```python
from build123d import *

# Parameters (mm, degrees)
EXTRUDE_1_DEPTH     = 5
CUT_EXTRUDE_1_DEPTH = 5
SKETCH_3_R          = 1.65
CUT_EXTRUDE_2_DEPTH = 10
SKETCH_4_R          = 11.2
SKETCH_4_R_2        = 11
SKETCH_4_R_3        = 1.65
SKETCH_4_R_4        = 1.6
CUT_EXTRUDE_3_DEPTH = 10
FILLET_1_R          = 15


with BuildPart() as part:
    # 草图1 → 凸台-拉伸1 (new body)
    with BuildSketch(Plane.XY):
        Polygon((65, 65), (65, 0), (195, 0), (195, 65), (260, 65), (260, 195), (195, 195), (195, 260), (65, 260), (65, 195), (0, 195), (0, 65), align=None)
    extrude(amount=EXTRUDE_1_DEPTH)

    # 草图2 → 切除-拉伸1 (cut)
    with BuildSketch(Plane(origin=(0, 0, 0), x_dir=(-1, 0, 0), z_dir=(0, 0, -1))):
        with BuildLine():
            Line((-106.8, 12.1), (-77, 12.1))
            ThreePointArc((-77, 12.1), (-74.9, 10), (-77, 7.9))
            Line((-77, 7.9), (-106.8, 7.9))
            ThreePointArc((-106.8, 7.9), (-108.9, 10), (-106.8, 12.1))
        make_face()
        with BuildLine():
            Line((-106.8, 42.1), (-77, 42.1))
            ThreePointArc((-77, 42.1), (-74.9, 40), (-77, 37.9))
            Line((-77, 37.9), (-106.8, 37.9))
            ThreePointArc((-106.8, 37.9), (-108.9, 40), (-106.8, 42.1))
        make_face()
        with BuildLine():
            Line((-153.2, 12.1), (-183, 12.1))
            ThreePointArc((-183, 12.1), (-185.1, 10), (-183, 7.9))
            Line((-183, 7.9), (-153.2, 7.9))
            ThreePointArc((-153.2, 7.9), (-151.1, 10), (-153.2, 12.1))
        make_face()
        with BuildLine():
            Line((-153.2, 42.1), (-183, 42.1))
            ThreePointArc((-183, 42.1), (-185.1, 40), (-183, 37.9))
            Line((-183, 37.9), (-153.2, 37.9))
            ThreePointArc((-153.2, 37.9), (-151.1, 40), (-153.2, 42.1))
        make_face()
        with BuildLine():
            Line((-106.8, 247.9), (-77, 247.9))
            ThreePointArc((-77, 247.9), (-74.9, 250), (-77, 252.1))
            Line((-77, 252.1), (-106.8, 252.1))
            ThreePointArc((-106.8, 252.1), (-108.9, 250), (-106.8, 247.9))
        make_face()
        with BuildLine():
            Line((-106.8, 217.9), (-77, 217.9))
            ThreePointArc((-77, 217.9), (-74.9, 220), (-77, 222.1))
            Line((-77, 222.1), (-106.8, 222.1))
            ThreePointArc((-106.8, 222.1), (-108.9, 220), (-106.8, 217.9))
        make_face()
        with BuildLine():
            Line((-153.2, 247.9), (-183, 247.9))
            ThreePointArc((-183, 247.9), (-185.1, 250), (-183, 252.1))
            Line((-183, 252.1), (-153.2, 252.1))
            ThreePointArc((-153.2, 252.1), (-151.1, 250), (-153.2, 247.9))
        make_face()
        with BuildLine():
            Line((-153.2, 217.9), (-183, 217.9))
            ThreePointArc((-183, 217.9), (-185.1, 220), (-183, 222.1))
            Line((-183, 222.1), (-153.2, 222.1))
            ThreePointArc((-153.2, 222.1), (-151.1, 220), (-153.2, 217.9))
        make_face()
    extrude(amount=-CUT_EXTRUDE_1_DEPTH, mode=Mode.SUBTRACT)

    # 草图3 → 切除-拉伸2 (cut)
    with BuildSketch(Plane.XY.offset(5)):
        with Locations((250, 185)):
            Circle(SKETCH_3_R)
        with Locations((250, 75)):
            Circle(SKETCH_3_R)
        with Locations((10, 75)):
            Circle(SKETCH_3_R)
        with Locations((10, 185)):
            Circle(SKETCH_3_R)
        with Locations((130, 75)):
            Circle(SKETCH_3_R)
        with Locations((130, 185)):
            Circle(SKETCH_3_R)
    extrude(amount=-CUT_EXTRUDE_2_DEPTH, mode=Mode.SUBTRACT)

    # 草图4 → 切除-拉伸3 (cut)
    with BuildSketch(Plane.XY.offset(5)):
        with Locations((80, 130)):
            Circle(SKETCH_4_R)
        with Locations((225, 130)):
            Circle(SKETCH_4_R_2)
        with Locations((190.7, 134.95)):
            Circle(SKETCH_4_R_3)
        with Locations((190.7, 125.05)):
            Circle(SKETCH_4_R_3)
        with Locations((239.3, 134.95)):
            Circle(SKETCH_4_R_3)
        with Locations((239.3, 125.05)):
            Circle(SKETCH_4_R_3)
        with Locations((64.5, 145.5)):
            Circle(SKETCH_4_R_4)
        with Locations((95.5, 145.5)):
            Circle(SKETCH_4_R_4)
        with Locations((95.5, 114.5)):
            Circle(SKETCH_4_R_4)
        with Locations((64.5, 114.5)):
            Circle(SKETCH_4_R_4)
        with Locations((193.180194847, 161.819805153)):
            Circle(SKETCH_4_R_4)
        with Locations((193.180194847, 98.180194847)):
            Circle(SKETCH_4_R_4)
        with Locations((115, 130)):
            Circle(SKETCH_4_R_4)
        with Locations((80, 95)):
            Circle(SKETCH_4_R_4)
        with Locations((45, 130)):
            Circle(SKETCH_4_R_4)
        with Locations((80, 165)):
            Circle(SKETCH_4_R_4)
        with Locations((225, 175)):
            Circle(SKETCH_4_R_4)
        with Locations((225, 85)):
            Circle(SKETCH_4_R_4)
        with Locations((256.819805153, 98.180194847)):
            Circle(SKETCH_4_R_4)
        with Locations((256.819805153, 161.819805153)):
            Circle(SKETCH_4_R_4)
    extrude(amount=-CUT_EXTRUDE_3_DEPTH, mode=Mode.SUBTRACT)

    # 圆角1
    fillet_1_edges = [part.edges().sort_by_distance(p)[0] for p in [
        (65, 0, 2.5),
        (65, 65, 2.5),
        (0, 65, 2.5),
        (0, 195, 2.5),
        (65, 195, 2.5),
        (65, 260, 2.5),
        (195, 260, 2.5),
        (195, 195, 2.5),
        (260, 195, 2.5),
        (260, 65, 2.5),
        (195, 65, 2.5),
        (195, 0, 2.5),
    ]]
    fillet(fillet_1_edges, radius=FILLET_1_R)


solid = part.part
```
Here's how the part is built. I have some questions about the finished solid (model axes, mm). Give positions to 0.01 mm unless a question says otherwise; leave off trailing zeros. Write each loop counter-clockwise with the first axis right and the second up, starting at its lowest first coordinate (ties: lowest second). Pieces come first, ordered by that corner, then holes.
(1) Thinking about a two-plate mould opening in X: for faces 1 (the face through (199.28, 60.49, 2.54)), 2 (the face through (71.745, 137.569, 2.535)), 3 (the face through (128, 132, 0)), which applies, pulls with the +X half, pulls with the -X half, needs draft (parallel to the pull), parting line crosses it, or undercut?
Output values:
face 1: pulls with the +X half
face 2: undercut
face 3: needs draft
(2) Imagine slicing it at B-B, the plane y = 191. Write out the boundary of the cut face in (x, z), and give its area (3 significant figures).
Output values:
outline: (4.8, 0) - (255.2, 0) - (255.2, 5) - (4.8, 5) - close
area: 1,250 mm2
(3) Imagine slicing it at A-A, the plane x = 204. Write out the boundary of the cut face in (y, z), and give its area (3 significant figures).
Output values:
outline: (63.75, 0) - (196.25, 0) - (196.25, 5) - (63.75, 5) - close
area: 663 mm2
(4) Imagine slicing it at C-C, the plane z = 1.45. Count the separate pieces of the cut face and the enclosed holes in it, and give its area (3 significant figures).
Output values:
separate pieces: 1
enclosed holes: 34
area: 48,400 mm2
(5) Will these pins go through, and if not, where does the flat tip stop? pin 1 (3 mm diameter, centred on y = 70.5, z = 4.5, fed in from -X); pin 2 (2.5 mm diameter, centred on y = 228, z = 3.5, fed in from -X).
Output values:
pin 1: stops at x = 2.31
pin 2: stops at x = 65
(6) If I drill on L1, parallel to X at y = 114.5, z = 2.15; L2, parallel to Y at x = 224, z = 1.45; L3, parallel to X at y = 185, z = 1.3, over which ranges is the centre line in solid material (lowest first)?
Output values:
L1: x = 0 to 62.9, 66.1 to 93.9, 97.1 to 260
L2: y = 65 to 83.75, 86.25 to 119.05, 140.95 to 173.75, 176.25 to 195
L3: x = 0.86 to 8.35, 11.65 to 128.35, 131.65 to 248.35, 251.65 to 259.14
